Autodesk Inventor part; units mm, degrees
ref_plane "YZ Plane" through (0, 0, 0) normal (1, 0, 0) x (0, 1, 0)
ref_plane "XZ Plane" through (0, 0, 0) normal (0, 1, 0) x (-1, 0, 0)
ref_plane "XY Plane" through (0, 0, 0) normal (0, 0, 1) x (1, 0, 0)
sketch "Náčrt1" plane through (0, 0, 0) normal (1, 0, 0) x (0, 1, 0)
  circle A0 centre (60, 0) radius 16
  circle A1 centre (60, 0) radius 30
  line L0 (0, 30) -> (0, -30)
  line L1 (0, -30) -> (60, -30)
  line L2 (0, 30) -> (60, 30)
  line L3 (0, 30) -> (0, 68)
  line L4 (0, 68) -> (12, 68)
  line L5 (12, 68) -> (12, 64)
  line L6 (12, 64) -> (75.4986, 25.6864)
  line L7 (0, 68) -> (-12, 68)
  line L8 (-12, 68) -> (-12, 30)
  line L9 (-12, 30) -> (-28, 30)
  line L10 (-28, 30) -> (-28, 20)
  line L11 (-28, 20) -> (-14, 20)
  line L12 (-14, 20) -> (-14, -20)
  line L13 (-14, -20) -> (-28, -20)
  line L14 (-28, -20) -> (-28, -30)
  line L15 (-28, -30) -> (0, -30)
  line L16 (0, 30) -> (-12, 30)
  point P0 (0, 0)
  dimension "d0" = 32
  dimension "d1" = 60
  dimension "d2" = 12
  dimension "d3" = 31.106
  dimension "d4" = 60
  dimension "d5" = 38
  dimension "d6" = 10
  dimension "d7" = 50
  dimension "d8" = 24
  dimension "d9" = 26
  dimension "d10" = 40
  dimension "d11" = 60.9972
  dimension "d12" = 30
  dimension "d13" = 12
extrude "Vysunutí1" add sketch "Náčrt1" against normal blind 34 contours A1
extrude "Vysunutí2" add sketch "Náčrt1" against normal blind 4 contours A1 L2 L3 L4 L5 L6
extrude "Vysunutí3" add sketch "Náčrt1" against normal blind 30 contours L1 L0 L2 A1
extrude "Vysunutí4" add sketch "Náčrt1" against normal blind 16 contours L16 L8 L7 L3
extrude "Vysunutí5" add sketch "Náčrt1" against normal blind 30 contours L15 L14 L13 L12 L11 L10 L9 L16 L0
extrude "Vysunutí6" add sketch "Náčrt1" along normal blind 34 contours A1
extrude "Vysunutí7" add sketch "Náčrt1" along normal blind 30 contours L1 L0 L2 A1
extrude "Vysunutí8" add sketch "Náčrt1" along normal blind 4 contours A1 L2 L3 L4 L5 L6
extrude "Vysunutí9" add sketch "Náčrt1" along normal blind 16 contours L16 L8 L7 L3
extrude "Vysunutí10" add sketch "Náčrt1" along normal blind 90 contours L15 L14 L13 L12 L11 L10 L9 L16 L0
sketch "Náčrt2" plane through (-16, -12, 30) normal (0, -1, 0) x (1, 0, 0)
  circle A0 centre (16, 50) radius 16
  circle A1 centre (16, 50) radius 8
  line L0 (20, 38) -> (32, 38)
  line L1 (32, 38) -> (32, 50)
  line L2 (0, 38) -> (0, 50)
  line L3 (32, 38) -> (26.583, 38)
  line L4 (12, 38) -> (0, 38)
  line L5 (0, 38) -> (5.417, 38)
  point P0 (16, -30)
  dimension "d34" = 32
  dimension "d35" = 16
  dimension "d36" = 12
extrude "Vysunutí11" add sketch "Náčrt2" against normal blind 24 contours A0
extrude "Vysunutí12" add sketch "Náčrt2" against normal blind 12 contours L1 L0 A0 | A0 L4 L2
sketch "Náčrt3" plane through (30, 0, 30) normal (0, 1, 0) x (1, 0, 0)
  circle A0 centre (36, 30) radius 9
  point P0 (-30, 30)
  dimension "d41" = 18
extrude "Vysunutí13" cut sketch "Náčrt3" against normal blind 14
properties part number "6"
Check sheet for the modelled part. Datum: model origin and axes. Units: mm. A direction names the side the tool comes from. Round coordinates to 2 decimals unless told otherwise and drop trailing zeros. Order: outer loops, then holes, each group sorted by start corner. A loop starts at its lowest first (then second) coordinate and runs counter-clockwise, first axis right, second up. Notation, with made-up numbers: (82.5, 3.25) -> (123.5, 3.25) arc R16 ccw to (123.5, 24.25) -> close; hole circle Ø7 at (50.25, 0). An arc over 180 degrees is marked (long way). Use CSV: the item, a comma, the result in double quotes.
(1) Cross-section at C-C (y = -6). Record the boundary of the cut face in (x, z), and give its area (3 significant figures).
Worked out:
outline,"(-30, -30) -> (90, -30) -> (90, 30) -> (16, 30) -> (16, 80) arc R16 ccw to (-16, 80) -> (-16, 30) -> (-30, 30) -> close; hole circle Ø16 at (0, 80); hole circle Ø18 at (66, 0)"
area,"8,750 mm²"
(2) Cross-section at D-D (z = -14). Record the boundary of the cut face in (x, y), and give its area (3 significant figures).
Worked out:
outline,"(-34, 33.47) -> (-30, 33.47) -> (-30, -14) -> (90, -14) -> (90, 0) -> (30, 0) -> (30, 33.47) -> (34, 33.47) -> (34, 52.25) -> (-34, 52.25) -> close; (-34, 67.75) -> (34, 67.75) -> (34, 86.53) -> (-34, 86.53) -> close"
area,"6,240 mm²"
(3) Cross-section at B-B (z = 0). Record the boundary of the cut face in (x, y), and give its area (3 significant figures).
Worked out:
outline,"(-34, 30) -> (-30, 30) -> (-30, -14) -> (57, -14) -> (57, 0) -> (30, 0) -> (30, 30) -> (34, 30) -> (34, 44) -> (-34, 44) -> close; (-34, 76) -> (34, 76) -> (34, 90) -> (-34, 90) -> close; (75, -14) -> (90, -14) -> (90, 0) -> (75, 0) -> close"
area,"5,130 mm²"
(4) Cross-section at A-A (x = 66). Record the boundary of the cut face in (y, z), and give its area (3 significant figures).
Worked out:
outline,"(-28, -30) -> (0, -30) -> (0, -9) -> (-14, -9) -> (-14, -20) -> (-28, -20) -> close; (-28, 20) -> (-14, 20) -> (-14, 9) -> (0, 9) -> (0, 30) -> (-28, 30) -> close"
area,"868 mm²"
(5) Tool access check on faces 1 (the face through (53, 0, 0)), 2 (the face through (0, -12, 56)), 3 (the face through (4, 20, 41)), 4 (the face through (-4, 20, 41)). Record the directions out of +Z, -Z, +X, -X, +Y, -Y that give a thin tool (end or side, any length) a straight path to the whole face; none if there is none.
Worked out:
face 1,"+Z, -Z, +X"
face 2,"+Z, +X, -X, -Y"
face 3,"+X, +Y"
face 4,"-X, +Y"
(6) Material ranges on line 1 along Z through (x, y) = (-17, 60); line 2 along Z through (x, y) = (0, -1); line 3 along X through (y, z) = (77, -3), recorded low to high. Write a range as from..to.
Worked out:
line 1,"-30..-16, 16..30"
line 2,"-30..72, 88..96"
line 3,"-34..34"
(7) Depth check by flat-ended pin: pin 1 (1.5 mm diameter, centred on x = 61.5, y = -1, fed in from +Z); pin 2 (3.5 mm diameter, centred on x = 9, z = 62.5, fed in from +Y); pin 3 (1.5 mm diameter, centred on y = 11.5, z = 19.5, fed in from +X). Enter the tip coordinate at first touch or a pass-through.
Worked out:
pin 1,"z = 30"
pin 2,"y = 0"
pin 3,"x = 30"
(8) Draft check along Y on faces 5 (the face through (-0.476, 44.015, -0.703)), 6 (the face through (-0.056, 43.305, 45.111)), 7 (the face through (0.647, 2.499, 95.987)). Enter one of: pulls with the +Y half, pulls with the -Y half, needs draft (parallel to the pull), parting line crosses it, or undercut.
Worked out:
face 5,"undercut"
face 6,"pulls with the +Y half"
face 7,"needs draft"
